Read the model definition and answer for the solid it produces. Units are mm, in the model's axes. A direction names the side the tool comes from. Give positions to 0.01 mm unless a question says otherwise; leave off trailing zeros. Order: outer loops, then holes, each group sorted by start corner. A loop starts at its lowest first (then second) coordinate and runs counter-clockwise, first axis right, second up. Notation, with made-up numbers: (-29, 87.25) -> (0, 87.25) arc R15 cw to (0, 94.25) -> close; hole circle Ø4 at (-34, -22.5). An arc over 180 degrees is marked (long way). Use one line per item in the form item = value.
Autodesk Inventor part; units mm, degrees
ref_plane "Work Plane1" through (18.5, -18.65, -16.9) normal (1, 0, 0) x (0, 0, -1)
ref_plane "Work Plane2" through (4.95, -18.65, -16.9) normal (1, 0, 0) x (0, 0, -1)
ref_plane "YZ Plane" through (0, 0, 0) normal (1, 0, 0) x (0, 1, 0)
sketch "Sketch1" plane through (0, 0, 0) normal (0, 1, 0) x (-1, 0, 0)
  line L0 (19.75, 23.5) -> (-19.75, 23.5)
  line L1 (-19.75, 23.5) -> (-19.75, -23.5)
  line L2 (-19.75, -23.5) -> (19.75, -23.5)
  line L3 (19.75, -23.5) -> (19.75, 23.5)
  line L4 (0, -28.9451) -> (0, 30.9067)
  line L5 (30.9717, 0) -> (-30.2589, 0)
  point P0 (0, 0)
  dimension "d0" = 39.5
  dimension "d1" = 47
extrude "Extrusion1" add sketch "Sketch1" along normal blind 1.15
sketch "Sketch2" plane through (0, 0, 0) normal (0, 1, 0) x (-1, 0, 0)
  line L0 (-18.6, -22.35) -> (-18.6, -16.9)
  line L1 (-18.6, -16.9) -> (-19.75, -16.9)
  line L2 (-19.75, -16.9) -> (-19.75, -23.5)
  line L3 (-19.75, -23.5) -> (19.75, -23.5)
  line L4 (19.75, -23.5) -> (19.75, -22.35)
  line L5 (19.75, -22.35) -> (-18.6, -22.35)
  line L6 (19.75, -23.5) -> (19.75, 23.5)
  point P0 (0, 0)
  point P1 (19.75, -22.925)
  dimension "d7" = 6.6
  dimension "d9" = 1.15
extrude "Extrusion2" add sketch "Sketch2" against normal blind 18.65
chamfer "Chamfer1" distance 1.15 angle 45 1 edges at (-0.575, 0, -22.35) measured on face at (5.8167, -12.4333, -22.35)
chamfer "Chamfer3" distance 1.75 angle 45 1 edges at (0, 1.15, -23.5)
sketch "Sketch3" plane through (19.75, -18.65, -23.5) normal (0, 0, -1) x (-1, 0, 0)
  line L0 (36.4, 8) -> (17.9, 8)
  line L1 (17.9, 8) -> (17.9, 15.2)
  line L2 (17.9, 15.2) -> (33.2, 15.2)
  line L3 (36.4, 12) -> (36.4, 8)
  circle A0 centre (5.5, 5.5) radius 1.35
  line L4 (33.2, 15.2) -> (36.4, 12)
  line L5 (0, 0) -> (0, 18.05)
  line L6 (39.5, 0) -> (0, 0)
  line L7 (39.5, 0) -> (39.5, 18.05)
  point P0 (19.75, 18.65)
  dimension "d19" = 2.7
  dimension "d21" = 135
  dimension "d22" = 135
  dimension "d24" = 18.5
  dimension "d25" = 7.2
  dimension "d34" = 5.5
  dimension "d35" = 5.5
  dimension "d36" = 8
  dimension "d43" = 3.1
  dimension "d47" = 4
extrude "Extrusion3" cut sketch "Sketch3" against normal blind 1.15
chamfer "Chamfer4" distance 2 angle 45 1 edges at (19.175, 0, -16.9)
chamfer "Chamfer5" distance 1.5 distance2 0.75 1 edges at (15.6, -13.15, -23.5) measured on face at (11.7904, -5.3126, -23.5)
fillet "Fillet1" radius 0.5 5 edges at (-16.65, -10.65, -22.925) (-16.65, -6.65, -22.925) (-13.45, -3.45, -22.925) (1.85, -10.65, -22.925) (1.85, -3.45, -22.925)
ref_plane "Work Plane1" through (18.5, -18.65, -16.9) normal (1, 0, 0) x (0, 0, -1)
sketch "Sketch5" plane through (18.5, -18.65, -16.9) normal (1, 0, 0) x (0, 0, -1)
  line L0 (-40.4, 18.65) -> (-2, 18.65)
  line L1 (-25.55, 18.65) -> (-28.55, 18.65)
  line L2 (-28.55, 18.65) -> (-28.55, 17.15)
  line L3 (-25.55, 16.15) -> (-25.55, 18.65)
  line L4 (-25.55, 16.15) -> (-30.35, 16.15)
  line L5 (-30.35, 16.15) -> (-30.35, 17.15)
  line L6 (-30.35, 17.15) -> (-28.55, 17.15)
  line L7 (5.45, 17.5) -> (5.45, 0)
  point P0 (-16.9, 18.65)
  dimension "d52" = 4.8
  dimension "d55" = 1.5
  dimension "d57" = 31
  dimension "d58" = 3
  dimension "d70" = 2.5
extrude "Extrusion4" add sketch "Sketch5" against normal blind 3
ref_plane "Work Plane2" through (4.95, -18.65, -16.9) normal (1, 0, 0) x (0, 0, -1)
sketch "Sketch6" plane through (4.95, -18.65, -16.9) normal (1, 0, 0) x (0, 0, -1)
  line L0 (4.3, 18.65) -> (-40.4, 18.65)
  line L1 (-4.05, 18.65) -> (-4.05, 16.15)
  line L2 (-4.05, 16.15) -> (-9.05, 16.15)
  line L3 (-9.05, 16.15) -> (-9.05, 17.25)
  line L4 (-9.05, 17.25) -> (-7.05, 17.25)
  line L5 (-7.05, 17.25) -> (-7.05, 18.65)
  line L6 (5.45, 17.5) -> (5.45, 0)
  point P0 (-16.9, 18.65)
  dimension "d62" = 5
  dimension "d63" = 2
  dimension "d64" = 2.5
  dimension "d68" = 9.5
  dimension "d69" = 1.4
extrude "Extrusion5" add sketch "Sketch6" against normal blind 4.75
fillet "Fillet4" radius 0.5 27 edges at (18.5, -2.5, 11.05) (15.5, -2.5, 11.05) (18.5, -0.75, 11.65) (17, 0, 11.65) (18.5, 0, 10.15) (18.5, -1.25, 8.65) (17, 0, 8.65) (17, -2.5, 8.65) (15.5, -1.25, 8.65) (15.5, 0, 10.15) (15.5, -0.75, 11.65) (15.5, -1.5, 12.55) (18.5, -1.5, 12.55) (17, -1.5, 11.65) (4.95, -0.7, -9.85) (4.95, 0, -11.35) (2.575, 0, -9.85) (4.95, -1.4, -8.85) (0.2, -1.4, -8.85) (0.2, -0.7, -9.85) (0.2, 0, -11.35) (0.2, -2.5, -10.35) (4.95, -2.5, -10.35) (2.575, -2.5, -12.85) (0.2, -1.25, -12.85) (2.575, 0, -12.85) (4.95, -1.25, -12.85)
properties part number "laptop_port_cover"
Item 1: The part is cut by section B-B on y = -13.15. Give the vertices of the cut face in (x, z), and give its area (3 significant figures).
Checks:
outline = (-19.75, -23.5) -> (11.4, -23.5) -> (12.9, -22.75) -> (12.9, -22.35) -> (-19.75, -22.35) -> close; (15.6, -22.75) -> (17.1, -23.5) -> (19.75, -23.5) -> (19.75, -16.9) -> (18.6, -16.9) -> (18.6, -22.35) -> (15.6, -22.35) -> close
area = 47.5 mm²
Item 2: Which of the six approach directions +Z, -Z, +X, -X, +Y, -Y give full straight-line access (tool end or side, diameter ignored) to faces 4 (the flat face through (-16.65, -8, -23)), 5 (the flat face through (17, -1, 8.65)), 6 (the flat face through (-0.8, -0.6, -21.8))?
Checks:
face_4 = +Z, -Z
face_5 = +X, -X, -Y
face_6 = -X, -Y
Item 3: The part is cut by section D-D on z = -11. Give the vertices of the cut face in (x, y), and give its area (3 significant figures).
Checks:
outline = (-19.75, 0) -> (-0.3, 0) arc R0.5 cw to (0.2, -0.5) -> (0.2, -2) arc R0.5 ccw to (0.7, -2.5) -> (4.45, -2.5) arc R0.5 ccw to (4.95, -2) -> (4.95, -0.5) arc R0.5 cw to (5.45, 0) -> (19.75, 0) -> (19.75, 1.15) -> (-19.75, 1.15) -> close
area = 57.3 mm²
Item 4: Straight lines are drawn through the part: L1, parallel to Z at x = 4, y = -17; L2, parallel to Y at x = 0, z = -18.5; L3, parallel to Y at x = 14.25, z = -22.55. For each, find the intervals that lie inside material, in ascending order. Write a range as from..to.
Checks:
L1 = -23.5..-22.35
L2 = 0..1.15
L3 = -18.65..-14.5, -11.8..0.35
Item 5: Determine the mould class of faces 1 (the flat face through (0.3, 0.3, -22.6)), 2 (the flat face through (-8, -10.65, -23)), 3 (the flat face through (19.75, -6.6, -17.3)) for opening direction Y: +Y half, -Y half, draft (parallel to the pull), parting line (faces both ways), or undercut.
Checks:
face_1 = +Y half
face_2 = undercut
face_3 = draft
Item 6: The part is cut by section C-C on x = 2.5. Give the vertices of the cut face in (y, z), and give its area (3 significant figures).
Checks:
outline = (-18.65, -23.5) -> (-0.6, -23.5) -> (1.15, -21.75) -> (1.15, 23.5) -> (0, 23.5) -> (0, -9.35) arc R0.5 cw to (-0.5, -9.85) -> (-1.4, -9.85) -> (-1.4, -7.85) -> (-2.5, -7.85) -> (-2.5, -12.35) arc R0.5 ccw to (-2, -12.85) -> (-0.5, -12.85) arc R0.5 cw to (0, -13.35) -> (0, -21.2) -> (-1.15, -22.35) -> (-18.65, -22.35) -> close
area = 84.4 mm²
Item 7: Given pin 1 Ø4.5 at (x, y) = (14.25, -13.15) entering from +Z; pin 2 Ø8 at (x, z) = (11, 1) entering from -Y; pin 3 Ø9 at (x, y) = (0, -6.5) entering from +Z, each flat-ended and moving along its own axis, determine where each tip first touches the part or whether it passes through.
Checks:
pin_1 = -22.35
pin_2 = 0
pin_3 = -7.85
Item 8: The part is cut by section A-A on x = -3.5. Give the vertices of the cut face in (y, z).
Checks:
outline = (-18.65, -23.5) -> (-10.65, -23.5) -> (-10.65, -22.35) -> (-18.65, -22.35) -> close; (-3.45, -23.5) -> (-0.6, -23.5) -> (1.15, -21.75) -> (1.15, 23.5) -> (0, 23.5) -> (0, -21.2) -> (-1.15, -22.35) -> (-3.45, -22.35) -> close
